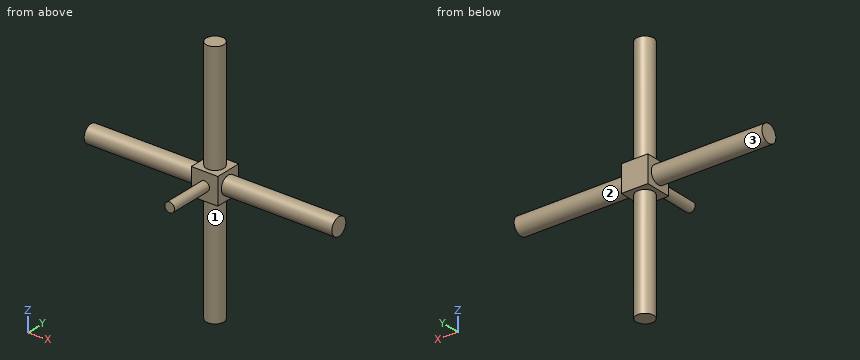
from build123d import *

# Parameters (mm, degrees)
SKETCH1_W           = 60
SKETCH1_H           = 60
BOSS_EXTRUDE1_DEPTH = 60
SKETCH2_R           = 20
BOSS_EXTRUDE2_DEPTH = 250
SKETCH3_R           = 20
BOSS_EXTRUDE3_DEPTH = 250
BOSS_EXTRUDE4_START = 250
SKETCH4_R           = 20
BOSS_EXTRUDE4_DEPTH = 250
BOSS_EXTRUDE5_START = 250
SKETCH5_R           = 20
BOSS_EXTRUDE5_DEPTH = 250
SKETCH6_R           = 11
BOSS_EXTRUDE6_DEPTH = 100


with BuildPart() as part:
    # Sketch1 → Boss-Extrude1 (new body)
    with BuildSketch(Plane(origin=(0, 0, 0), x_dir=(1, 0, 0), z_dir=(0, 1, 0))):
        Rectangle(SKETCH1_W, SKETCH1_H)
    extrude(amount=BOSS_EXTRUDE1_DEPTH)

    # Sketch2 → Boss-Extrude2 (add)
    with BuildSketch(Plane.XY.offset(30)):
        with Locations((0, 30)):
            Circle(SKETCH2_R)
    extrude(amount=BOSS_EXTRUDE2_DEPTH)

    # Sketch3 → Boss-Extrude3 (add)
    with BuildSketch(Plane.ZY.offset(30)):
        with Locations((0, 30)):
            Circle(SKETCH3_R)
    extrude(amount=BOSS_EXTRUDE3_DEPTH)

    # Sketch4 → Boss-Extrude4 (add)
    with BuildSketch(Plane(origin=(0, 0, -30), x_dir=(-1, 0, 0), z_dir=(0, 0, -1)).offset(BOSS_EXTRUDE4_START)):
        with Locations(Location((0, 30, 0), (0, 0, 180))):
            Circle(SKETCH4_R)
    extrude(amount=-BOSS_EXTRUDE4_DEPTH)

    # Sketch5 → Boss-Extrude5 (add)
    with BuildSketch(Plane(origin=(30, 0, 0), x_dir=(0, 0, -1), z_dir=(1, 0, 0)).offset(BOSS_EXTRUDE5_START)):
        with Locations(Location((0, 30, 0), (0, 0, 180))):
            Circle(SKETCH5_R)
    extrude(amount=-BOSS_EXTRUDE5_DEPTH)

    # Sketch6 → Boss-Extrude6 (add)
    with BuildSketch(Plane.XZ):
        with Locations(Location((0, 0, 0), (0, 0, 270))):
            Circle(SKETCH6_R)
    extrude(amount=BOSS_EXTRUDE6_DEPTH)


solid = part.part
The listing builds one solid part. Answer for the finished solid, in the listing's coordinates (mm). Face numbers are marked on the shaded views. A direction names the side the tool comes from. Round coordinates to 2 decimals unless told otherwise and drop trailing zeros. Write each loop counter-clockwise with the first axis right and the second up, starting at its lowest first coordinate (ties: lowest second). Pieces come first, ordered by that corner, then holes. Notation, with made-up numbers: M 82.5,-16.75 L 96.5,-16.75 A20 cw 96.5,4.25 Z; hole C -7,61 d11. An arc over 180 degrees is marked long. Write each question's results on one line, items separated by ' | '. Start each with the question number.
(1) Each of these flat-tipped pins is pushed along its axis until it touches: P1, Ø8, axis at y = 18.5, z = -77.5, coming from the +X side; P2, Ø8, axis at x = 212.5, y = 18, coming from the -Z side; P3, Ø2, axis at y = 14, z = 130.5, coming from the +X side. Where does it stop, or does it pass through?
(2) The part is cut by section A-A, the plane y = 30. Write down the section's boundary in (x, z), and give its area (3 significant figures).
(3) The part is cut by section B-B, the plane z = 0. Write down the section's boundary in (x, y), and give its area (3 significant figures).
(4) The part is cut by section D-D, the plane y = -46. Write down the section's boundary in (x, z), and give its area (3 significant figures).
(5) Find the intervals of material crossed by line 1 (Z direction, x = 22, y = 10.5); line 2 (X direction, y = -30, z = -1); line 3 (Y direction, x = -10.5, z = 142), in increasing order.
(6) The part is cut by section C-C, the plane x = -95. Write down the section's boundary in (y, z).
(7) For the marked faces 1, 2 and 3, determine the directions among +Z, -Z, +X, -X, +Y, -Y from which every point of the face is accessible in a straight line to the end or side of a thin tool.
Worked answers:
1) P1: stops at x = 18.54 | P2: stops at z = -18.33 | P3: stops at x = 13.23
2) outline: M -280,-20 L -30,-20 L -30,-30 L -20,-30 L -20,-280 L 20,-280 L 20,-30 L 30,-30 L 30,-20 L 280,-20 L 280,20 L 30,20 L 30,30 L 20,30 L 20,280 L -20,280 L -20,30 L -30,30 L -30,20 L -280,20 Z | area: 43,600 mm²
3) outline: M -280,10 L -30,10 L -30,0 L -11,0 L -11,-100 L 11,-100 L 11,0 L 30,0 L 30,10 L 280,10 L 280,50 L 30,50 L 30,60 L -30,60 L -30,50 L -280,50 Z | area: 25,800 mm²
4) outline: C 0,0 d22 | area: 380 mm²
5) line 1: z = -30 to 30 | line 2: x = -10.95 to 10.95 | line 3: y = 12.98 to 47.02
6) outline: C 30,0 d40
7) face 1: -Z | face 2: +X | face 3: -X
